from build123d import *

# Parameters (mm, degrees)
DODANIE_WYCI_GNI_CIE1_DEPTH = 702
SZKIC2_R                    = 6
DODANIE_WYCI_GNI_CIE2_DEPTH = 5
SZKIC4_R                    = 6
WYTNIJ_WYCI_GNI_CIE1_DEPTH  = 65


with BuildPart() as part:
    # Szkic1 → Dodanie-wyciągnięcie1 (new body)
    with BuildSketch(Plane.XY):
        with BuildLine():
            Line((0, 4), (0, 36))
            ThreePointArc((0, 36), (1.171572875, 38.828427125), (4, 40))
            Line((4, 40), (56, 40))
            ThreePointArc((56, 40), (58.828427125, 38.828427125), (60, 36))
            Line((60, 36), (60, 4))
            ThreePointArc((60, 4), (58.828427125, 1.171572875), (56, 0))
            Line((56, 0), (4, 0))
            ThreePointArc((4, 0), (1.171572875, 1.171572875), (0, 4))
        make_face()
        with BuildLine():
            Line((2, 4), (2, 36))
            ThreePointArc((2, 36), (2.585786438, 37.414213562), (4, 38))
            Line((4, 38), (56, 38))
            ThreePointArc((56, 38), (57.414213562, 37.414213562), (58, 36))
            Line((58, 36), (58, 4))
            ThreePointArc((58, 4), (57.414213562, 2.585786438), (56, 2))
            Line((56, 2), (4, 2))
            ThreePointArc((4, 2), (2.585786438, 2.585786438), (2, 4))
        make_face(mode=Mode.SUBTRACT)
    extrude(amount=DODANIE_WYCI_GNI_CIE1_DEPTH)

    # Szkic2 → Dodanie-wyciągnięcie2 (add)
    with BuildSketch(Plane(origin=(0, 40, 0), x_dir=(1, 0, 0), z_dir=(0, 1, 0))):
        Polygon((0, 0), (-50, 0), (-50, -40), (110, -40), (110, 0), align=None)
        with Locations(Location((-25, -20, 0), (0, 0, 270))):
            Circle(SZKIC2_R, mode=Mode.SUBTRACT)
        with Locations(Location((85, -20, 0), (0, 0, 270))):
            Circle(SZKIC2_R, mode=Mode.SUBTRACT)
    dodanie_wyci_gni_cie2 = extrude(amount=DODANIE_WYCI_GNI_CIE2_DEPTH)

    # Lustro1: Dodanie-wyciągnięcie2 across plane
    add(dodanie_wyci_gni_cie2.mirror(Plane(origin=(0, 0, 351), x_dir=(1, 0, 0), z_dir=(0, 0, -1))))

    # Szkic4 → Wytnij-wyciągnięcie1 (cut)
    with BuildSketch(Plane(origin=(60, 0, 0), x_dir=(0, 0, -1), z_dir=(1, 0, 0))):
        with Locations((-101, 20)):
            Circle(SZKIC4_R)
        with Locations((-351, 20)):
            Circle(SZKIC4_R)
        with Locations((-601, 20)):
            Circle(SZKIC4_R)
    extrude(amount=-WYTNIJ_WYCI_GNI_CIE1_DEPTH, mode=Mode.SUBTRACT)


solid = part.part
The listing builds one solid part. Answer for the finished solid, in the listing's coordinates (mm). A direction names the side the tool comes from. Give positions to 0.01 mm unless a question says otherwise; leave off trailing zeros. Order: outer loops, then holes, each group sorted by start corner. A loop starts at its lowest first (then second) coordinate and runs counter-clockwise, first axis right, second up. Notation, with made-up numbers: (72.25, 35.25) - (129.25, 35.25) arc R19 ccw to (129.25, 47.25) - close; hole circle Ø10 at (13, -7.5). An arc over 180 degrees is marked (long way). Answer as CSV lines item,"result".
Q1. A cutting plane is placed at C-C, the plane z = 351. Determine the outline of the cut face in (x, y).
Answer key:
outline,"(0, 4) arc R4 ccw to (4, 0) - (56, 0) arc R4 ccw to (60, 4) - (60, 14) - (58, 14) - (58, 4) arc R2 cw to (56, 2) - (4, 2) arc R2 cw to (2, 4) - (2, 14) - (0, 14) - close; (0, 26) - (2, 26) - (2, 36) arc R2 cw to (4, 38) - (56, 38) arc R2 cw to (58, 36) - (58, 26) - (60, 26) - (60, 36) arc R4 ccw to (56, 40) - (4, 40) arc R4 ccw to (0, 36) - close"
Q2. A cutting plane is placed at A-A, the plane z = 20. Determine the outline of the cut face in (x, y), and give its area (3 significant figures).
Answer key:
outline,"(-50, 40) - (-31, 40) - (-31, 45) - (-50, 45) - close; (-19, 40) - (4, 40) arc R4 ccw to (0, 36) - (0, 4) arc R4 ccw to (4, 0) - (56, 0) arc R4 ccw to (60, 4) - (60, 36) arc R4 ccw to (56, 40) - (79, 40) - (79, 45) - (-19, 45) - close; (91, 40) - (110, 40) - (110, 45) - (91, 45) - close; hole (2, 4) arc R2 ccw to (4, 2) - (56, 2) arc R2 ccw to (58, 4) - (58, 36) arc R2 ccw to (56, 38) - (4, 38) arc R2 ccw to (2, 36) - close"
area,"1,050 mm^2"
Q3. Straight lines are drawn through the part: L1, parallel to X at y = 41.55, z = 682; L2, parallel to X at y = 23.5, z = 577; L3, parallel to Y at x = 14, z = 147. For each, find the intervals that lie inside material, in ascending order.
Answer key:
L1,"x = -50 to -31, -19 to 79, 91 to 110"
L2,"x = 0 to 2, 58 to 60"
L3,"y = 0 to 2, 38 to 40"
Q4. A cutting plane is placed at D-D, the plane x = 97.5. Determine the outline of the cut face in (y, z).
Answer key:
outline,"(40, 0) - (45, 0) - (45, 40) - (40, 40) - close; (40, 662) - (45, 662) - (45, 702) - (40, 702) - close"
Q5. Which of the six approach directions +Z, -Z, +X, -X, +Y, -Y give full straight-line access (tool end or side, diameter ignored) to faces 1 (the face through (59, 20, 607)), 2 (the face through (30, 38, 346)), 3 (the face through (30, 40, 347))?
Answer key:
face 1,"+X, -X"
face 2,"+Z, -Z"
face 3,"+X, -X, +Y"
Q6. Determine the mould class of faces 4 (the face through (59.014, 21.802, 345.277)), 5 (the face through (24, 39, 702)), 6 (the face through (-27.3, 42.46, 25.54)), 7 (the face through (30, 2, 346)) for opening direction Z: pulls with the +Z half, pulls with the -Z half, needs draft (parallel to the pull), parting line crosses it, or undercut.
Answer key:
face 4,"undercut"
face 5,"pulls with the +Z half"
face 6,"undercut"
face 7,"needs draft"
Q7. A cutting plane is placed at B-B, the plane y = 20. Count the separate pieces of the cut face and the enclosed holes in it, and give its area (3 significant figures).
Answer key:
separate pieces,"8"
enclosed holes,"0"
area,"2,660 mm^2"
Q8. Each of these flat-tipped pins is pushed along its axis until it touches: pin 1 Ø9.5 at (y, z) = (20, 351) entering from +X; pin 2 Ø9.5 at (y, z) = (19, 313) entering from +X; pin 3 Ø14 at (x, z) = (85, 20) entering from -Y; pin 4 Ø12 at (x, z) = (59.5, 280) entering from +Y. Where does it stop, or does it pass through?
Answer key:
pin 1,"passes through"
pin 2,"stops at x = 60"
pin 3,"stops at y = 40"
pin 4,"stops at y = 40"
